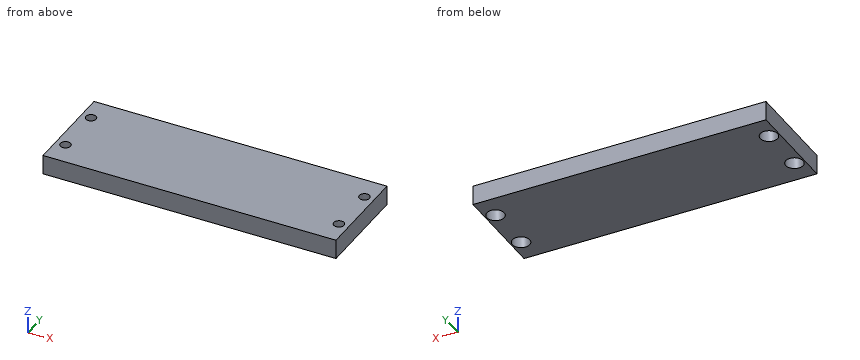
```python
from build123d import *

# Parameters (mm, degrees)
SKETCH_1_W             = 120
SKETCH_1_H             = 40
EXTRUDE_1_DEPTH        = 8
SKETCH_2_R             = 2.1
CUT_EXTRUDE_1_DEPTH    = 50
PATTERN_LINEAR_2_COUNT = 2
PATTERN_LINEAR_2_PITCH = 112
SKETCH_3_R             = 3.55
CUT_EXTRUDE_2_DEPTH    = 5


with BuildPart() as part:
    # Эскиз1 → Бобышка-Вытянуть1 (new body)
    with BuildSketch(Plane.XY):
        Rectangle(SKETCH_1_W, SKETCH_1_H)
    extrude(amount=EXTRUDE_1_DEPTH)

    # Эскиз2 → Вырез-Вытянуть1 (cut)
    with BuildSketch(Plane.XY.offset(8)):
        with Locations((-56, 10)):
            Circle(SKETCH_2_R)
        with Locations((-56, -10)):
            Circle(SKETCH_2_R)
    cut_extrude_1 = extrude(amount=-CUT_EXTRUDE_1_DEPTH, mode=Mode.SUBTRACT)

    # Линейный массив2: Вырез-Вытянуть1 ×2
    with Locations(*[(i * PATTERN_LINEAR_2_PITCH, 0, 0) for i in range(1, PATTERN_LINEAR_2_COUNT)]):
        add(cut_extrude_1, mode=Mode.SUBTRACT)

    # Эскиз3 → Вырез-Вытянуть2 (cut)
    with BuildSketch(Plane(origin=(0, 0, 0), x_dir=(-1, 0, 0), z_dir=(0, 0, -1))):
        with Locations((-56, 10)):
            Circle(SKETCH_3_R)
        with Locations((-56, -10)):
            Circle(SKETCH_3_R)
        with Locations((56, 10)):
            Circle(SKETCH_3_R)
        with Locations((56, -10)):
            Circle(SKETCH_3_R)
    extrude(amount=-CUT_EXTRUDE_2_DEPTH, mode=Mode.SUBTRACT)


solid = part.part
```
Read the model definition and answer for the solid it produces. Units are mm, in the model's axes. Give positions to 0.01 mm unless a question says otherwise; leave off trailing zeros. Write each loop counter-clockwise with the first axis right and the second up, starting at its lowest first coordinate (ties: lowest second). Pieces come first, ordered by that corner, then holes. Notation, with made-up numbers: M 82,-36 L 132,-36 A24 cw 132,-25 Z; hole C 64,-1 d11. An arc over 180 degrees is marked long. Put each result on its own line as item: value. Start each with the question number.
1. Consider line 1 along Y through (x, z) = (56, 2.25); line 2 along Y through (x, z) = (-56, 6.7); line 3 along X through (y, z) = (11, 5.5). Determine where each line is inside the solid, lowest interval first.
2. This flat-tipped pin is pushed along its axis until it touches: pin 1 Ø3.5 at (x, y) = (55, -9) entering from -Z. Where does it stop, or does it pass through?
3. The part is cut by section B-B, the plane x = 56. Give the vertices of the cut face in (y, z), and give its area (3 significant figures).
4. The part is cut by section A-A, the plane y = 10. Give the vertices of the cut face in (x, z).
Final values:
1. line 1: y = -20 to -13.55, -6.45 to 6.45, 13.55 to 20
1. line 2: y = -20 to -12.1, -7.9 to 7.9, 12.1 to 20
1. line 3: x = -60 to -57.85, -54.15 to 54.15, 57.85 to 60
2. pin 1: stops at z = 5
3. outline: M -20,0 L -13.55,0 L -13.55,5 L -12.1,5 L -12.1,8 L -20,8 Z; M -7.9,5 L -6.45,5 L -6.45,0 L 6.45,0 L 6.45,5 L 7.9,5 L 7.9,8 L -7.9,8 Z; M 12.1,5 L 13.55,5 L 13.55,0 L 20,0 L 20,8 L 12.1,8 Z
3. area: 224 mm²
4. outline: M -60,0 L -59.55,0 L -59.55,5 L -58.1,5 L -58.1,8 L -60,8 Z; M -53.9,5 L -52.45,5 L -52.45,0 L 52.45,0 L 52.45,5 L 53.9,5 L 53.9,8 L -53.9,8 Z; M 58.1,5 L 59.55,5 L 59.55,0 L 60,0 L 60,8 L 58.1,8 Z
